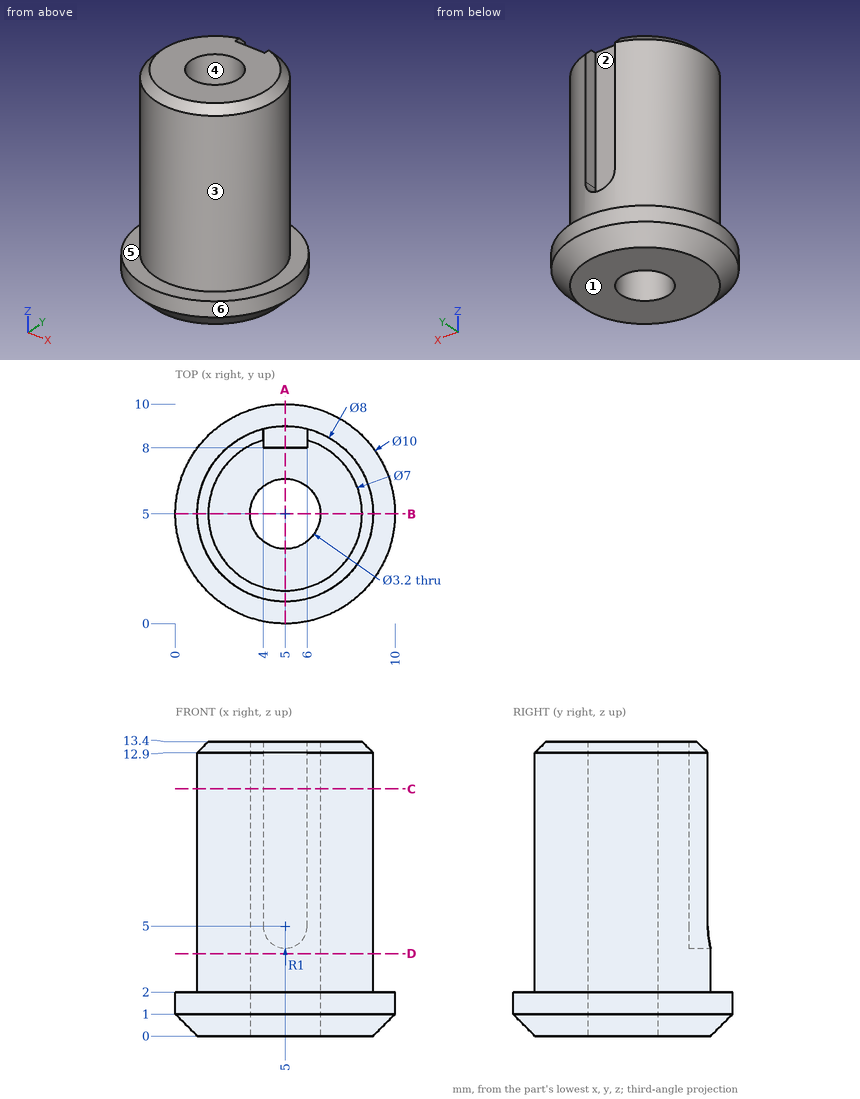
The figure shows three views and two pictorial views of one solid part (mm, origin at its lowest corner). Answer the questions. A direction names the side the tool comes from. Coordinates: 2 decimals unless noted, no trailing zeros. Write each loop counter-clockwise with the first axis right and the second up, starting at its lowest first coordinate (ties: lowest second). Pieces come first, ordered by that corner, then holes.
1. The part is cut by section A-A, the plane x = 5. Write down the section's boundary in (y, z).
Results list:
outline: (0, 1) - (1, 0) - (3.4, 0) - (3.4, 13.4) - (1.5, 13.4) - (1, 12.9) - (1, 2) - (0, 2) - close; (6.6, 0) - (9, 0) - (10, 1) - (10, 2) - (9, 2) - (9, 4) - (8, 4) - (8, 13.4) - (6.6, 13.4) - close
2. Consider line 1 along Y through (x, z) = (5, 8); line 2 along X through (y, z) = (5, 8.5). Determine where each line is inside the solid, lowest interval first.
Results list:
line 1: y = 1 to 3.4, 6.6 to 8
line 2: x = 1 to 3.4, 6.6 to 9
3. The part is cut by section B-B, the plane y = 5. Write down the section's boundary in (x, z).
Results list:
outline: (0, 1) - (1, 0) - (3.4, 0) - (3.4, 13.4) - (1.5, 13.4) - (1, 12.9) - (1, 2) - (0, 2) - close; (6.6, 0) - (9, 0) - (10, 1) - (10, 2) - (9, 2) - (9, 12.9) - (8.5, 13.4) - (6.6, 13.4) - close
4. For a pull along Y with two mould halves and no side action, classify the marked faces 4, 5 and 6 as +Y half, -Y half, draft (parallel to the pull), parting line (faces both ways), or undercut.
Results list:
face 4: undercut
face 5: draft
face 6: parting line
5. For the marked faces 1, 2 and 3, determine the directions among +Z, -Z, +X, -X, +Y, -Y from which every point of the face is accessible in a straight line to the end or side of a thin tool.
Results list:
face 1: -Z, +X, -X, +Y, -Y
face 2: +Z, +Y
face 3: +Z
6. Flat-ended cylindrical pins translate along their axes: pin 1 (1.9 mm diameter, centred on x = 5, y = 5, fed in from -Z); pin 2 (3 mm diameter, centred on x = 3, y = 4, fed in from -Z); pin 3 (3 mm diameter, centred on x = 5, z = 11, fed in from -Y); pin 4 (3 mm diameter, centred on y = 2, z = 9, fed in from +X). Find the tip coordinate at first contact, or state that the pin passes through.
Results list:
pin 1: passes through
pin 2: stops at z = 0
pin 3: stops at y = 1
pin 4: stops at x = 8.71
7. The part is cut by section C-C, the plane z = 11.25. Write down the section's boundary in (x, y), and give its area (3 significant figures).
Results list:
outline: (4, 8) - (4, 8.87) arc R4 ccw (long way) to (6, 8.87) - (6, 8) - close; hole circle Ø3.2 at (5, 5)
area: 40.3 mm2
8. The part is cut by section D-D, the plane z = 3.75. Write down the section's boundary in (x, y).
Results list:
outline: circle Ø8 at (5, 5); hole circle Ø3.2 at (5, 5)
